Read the model definition and answer for the solid it produces. Units are mm, in the model's axes. Face numbers are marked on the shaded views. A direction names the side the tool comes from. Round coordinates to 2 decimals unless told otherwise and drop trailing zeros. Write each loop counter-clockwise with the first axis right and the second up, starting at its lowest first coordinate (ties: lowest second). Pieces come first, ordered by that corner, then holes.
from build123d import *

# Parameters (mm, degrees)
SKETCH_11_W         = 24
SKETCH_11_H         = 40
SKETCH_11_W_2       = 13
SKETCH_11_H_2       = 23
EXTRUDE_1_DEPTH     = 4
SKETCH_12_R         = 1.5
CUT_EXTRUDE_1_DEPTH = 4
EXTRUDE_2_REACH     = 99.098
SKETCH_13_W         = 24
SKETCH_13_H         = 3.464101616
SKETCH_14_R         = 1.5
CUT_EXTRUDE_2_DEPTH = 4


with BuildPart() as part:
    # 草图11 → 凸台-拉伸1 (new body)
    with BuildSketch(Plane(origin=(0, 43, 74.478184725), x_dir=(-1, 0, 0), z_dir=(0, 0.500000000000001, 0.866025403784438))):
        with Locations((-0.009864086, -5.25)):
            Rectangle(SKETCH_11_W, SKETCH_11_H)
        with Locations((-0.009864086, -5.25)):
            Rectangle(SKETCH_11_W_2, SKETCH_11_H_2, mode=Mode.SUBTRACT)
    extrude(amount=EXTRUDE_1_DEPTH)

    # 草图12 → 切除-拉伸1 (cut)
    with BuildSketch(Plane(origin=(0, 43, 74.478184725), x_dir=(-1, 0, 0), z_dir=(0, -0.5000000000000009, -0.8660254037844383))):
        with Locations(Location((0, 19.1, 0), (0, 0, 90))):
            Circle(SKETCH_12_R)
        with Locations(Location((0, -8.6, 0), (0, 0, 90))):
            Circle(SKETCH_12_R)
    extrude(amount=-CUT_EXTRUDE_1_DEPTH, mode=Mode.SUBTRACT)

    # 凸台-拉伸2: up to this face of the body (flat: up to its plane)
    extrude_2_end = Plane(part.part.faces().sort_by_distance((0.009864086, 65.867141446, 63.585235533))[0])
    # 草图13 → 凸台-拉伸2 (add, up to the picked face)
    with BuildSketch(Plane(origin=(0, 75, 0), x_dir=(1, 0, 0), z_dir=(0, 1, 0)), mode=Mode.PRIVATE) as extrude_2_sk1:
        with Locations((0.009864086, -63.585235533)):
            Rectangle(SKETCH_13_W, SKETCH_13_H)
    extrude_2_tool1 = split(extrude(extrude_2_sk1.sketch, amount=-EXTRUDE_2_REACH, mode=Mode.PRIVATE), bisect_by=extrude_2_end, keep=Keep.BOTH, mode=Mode.PRIVATE)
    add(extrude_2_tool1.solids().sort_by(Axis((0.009864, 75, 63.585236), (0, -1, 0)))[0])

    # 草图14 → 切除-拉伸2 (cut)
    with BuildSketch(Plane(origin=(0, 0, 61.853184725), x_dir=(-1, 0, 0), z_dir=(0, 0, -1))):
        with Locations((8.990135914, 71)):
            Circle(SKETCH_14_R)
        with Locations((-9.009864086, 71)):
            Circle(SKETCH_14_R)
    extrude(amount=-CUT_EXTRUDE_2_DEPTH, mode=Mode.SUBTRACT)


solid = part.part
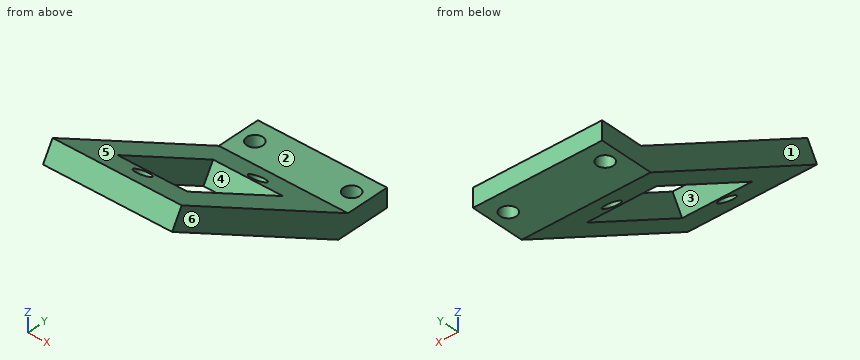
Q1. Section D-D (y = 43.5) is taken. Determine the outline of the cut face in (x, z).
Verdict:
outline: (-11.99, 74.19) - (-6.49, 74.19) - (-6.49, 78.81) - (-11.99, 78.81) - close; (6.51, 74.19) - (12.01, 74.19) - (12.01, 78.81) - (6.51, 78.81) - close
Q2. Straight lines are drawn through the part: probe 1 along X at (y, z) = (71, 64.35); probe 2 along X at (y, z) = (50.5, 72.5); probe 3 along Y at (x, z) = (1.75, 82.5). For each, find the intervals that lie inside material, in ascending order.
Verdict:
probe 1: x = -11.99 to -10.49, -7.49 to 7.51, 10.51 to 12.01
probe 2: x = -11.99 to -6.49, 6.51 to 12.01
probe 3: y = 30.6 to 37.11
Q3. Which of the six approach directions +Z, -Z, +X, -X, +Y, -Y give full straight-line access (tool end or side, diameter ignored) to the marked faces 1, 2 and 3?
Verdict:
face 1: +Z, -Z, -X, +Y, -Y
face 2: +Z, +X, -X, +Y
face 3: -Z, +Y
Q4. Flat-ended cylindrical pins translate along their axes: pin 1 Ø1.5 at (x, y) = (4.5, 60.5) entering from +Z; pin 2 Ø6.5 at (x, y) = (-4.5, 71.5) entering from +Z; pin 3 Ø12 at (x, y) = (7, 49.5) entering from -Z; pin 4 Ø2.5 at (x, y) = (-8.99, 71) entering from -Z. Find the tip coordinate at first contact, or state that the pin passes through.
Verdict:
pin 1: stops at z = 69.43
pin 2: stops at z = 65.32
pin 3: stops at z = 67.26
pin 4: passes through
Q5. Section B-B (y = 71) is taken. Determine the outline of the cut face in (x, z), then the cut area to 3 significant figures.
Verdict:
outline: (-11.99, 61.85) - (-10.49, 61.85) - (-10.49, 65.32) - (-11.99, 65.32) - close; (-7.49, 61.85) - (7.51, 61.85) - (7.51, 65.32) - (-7.49, 65.32) - close; (10.51, 61.85) - (12.01, 61.85) - (12.01, 65.32) - (10.51, 65.32) - close
area: 62.4 mm2
Q6. Section A-A (x = -3) is taken. Determine the outline of the cut face in (y, z).
Verdict:
outline: (30.23, 81.85) - (37.59, 77.6) - (39.59, 81.07) - (32.23, 85.32) - close; (57.51, 66.1) - (64.87, 61.85) - (75, 61.85) - (75, 65.32) - (66.87, 65.32) - (59.51, 69.57) - close
Q7. Section C-C (z = 75) is taken. Determine the outline of the cut face in (x, y), then the cut area to 3 significant figures.
Verdict:
outline: (-11.99, 42.1) - (-6.49, 42.1) - (-6.49, 50.1) - (-11.99, 50.1) - close; (6.51, 42.1) - (12.01, 42.1) - (12.01, 50.1) - (6.51, 50.1) - close
area: 88.0 mm2
Q8. Determine the mould class of the marked faces 4, 5 and 6 for opening direction X: pulls with the +X half, pulls with the -X half, needs draft (parallel to the pull), parting line crosses it, or undercut.
Verdict:
face 4: undercut
face 5: needs draft
face 6: pulls with the +X half
